Here's the drawing with two shaded views (mm, measured from the low corner). I have some questions. A direction names the side the tool comes from. Coordinates: 2 decimals unless noted, no trailing zeros. Write each loop counter-clockwise with the first axis right and the second up, starting at its lowest first coordinate (ties: lowest second). Pieces come first, ordered by that corner, then holes. Notation, with made-up numbers: (60, 40.5) -> (110, 40.5) arc R27 ccw to (110, 66.5) -> close; hole circle Ø3 at (30, 71). An arc over 180 degrees is marked (long way). Use one line per item in the form item = value.
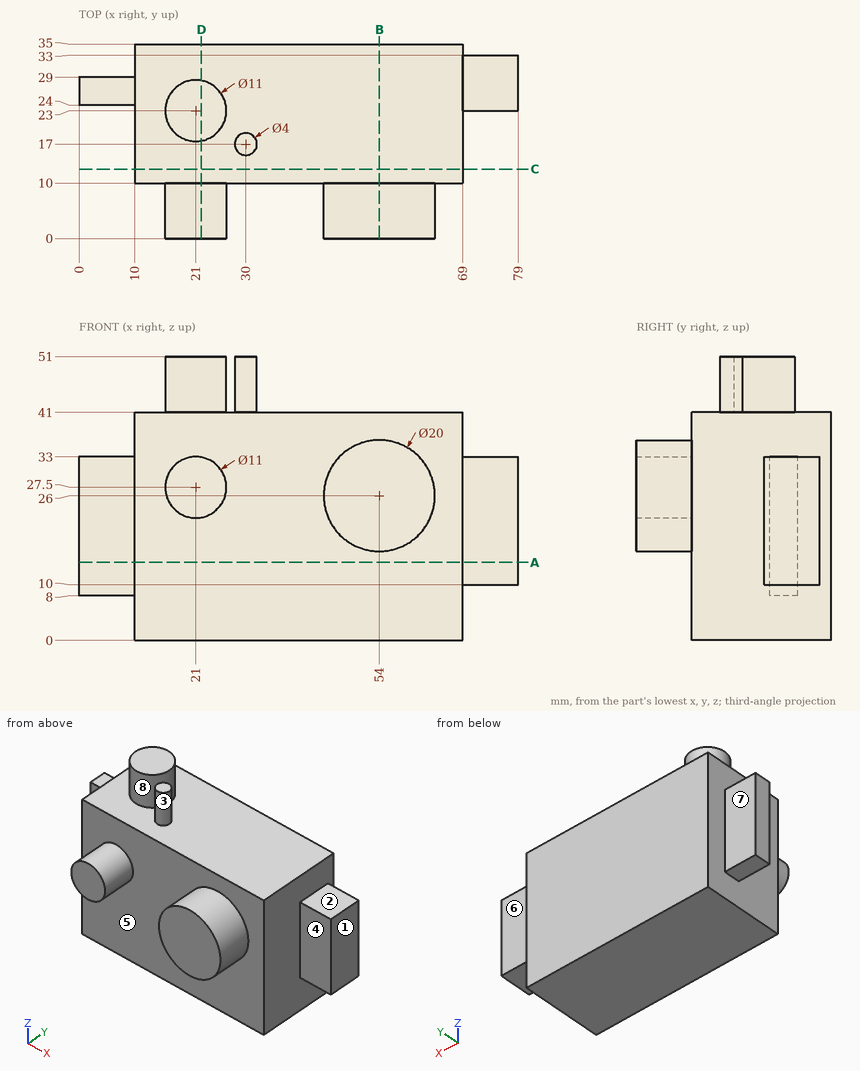
Q1. Suppose I cut it at B-B (x = 54). Write out the boundary of the cut face in (y, z), then the cut area to 4 significant figures.
Return value:
outline = (0, 16) -> (10, 16) -> (10, 0) -> (35, 0) -> (35, 41) -> (10, 41) -> (10, 36) -> (0, 36) -> close
area = 1,225 mm2
Q2. Suppose I cut it at A-A (z = 14). Write out the boundary of the cut face in (x, y).
Return value:
outline = (0, 24) -> (10, 24) -> (10, 10) -> (69, 10) -> (69, 23) -> (79, 23) -> (79, 33) -> (69, 33) -> (69, 35) -> (10, 35) -> (10, 29) -> (0, 29) -> close
Q3. Thinking about a two-plate mould opening in X: for the marked faces 1, 2 and 3, which applies, released by +X, released by -X, zero draft, split by the parting line, or undercut?
Return value:
face_1 = released by +X
face_2 = zero draft
face_3 = undercut
Q4. If I drill on line 1 (X direction, y = 19.5, z = 37.5); line 2 (Y direction, x = 28, z = 29.5); line 3 (Z direction, x = 11.5, y = 29), over which ranges is the centre line in solid material (lowest first)? Write a range as from..to.
Return value:
line_1 = 10..69
line_2 = 10..35
line_3 = 0..41
Q5. For the marked faces 4, 5, 6, 7 and 8, which set-ups out of +Z, -Z, +X, -X, +Y, -Y let a thin tool reach every point of the face, with its end or its side?
Return value:
face_4 = +Z, -Z, +X, -Y
face_5 = -Y
face_6 = +Z, -Z, +X, +Y
face_7 = +Z, -Z, -X, +Y
face_8 = +Z
Q6. Suppose I cut it at C-C (y = 12.5). Write out the boundary of the cut face in (x, z).
Return value:
outline = (10, 0) -> (69, 0) -> (69, 41) -> (10, 41) -> close
Q7. Suppose I cut it at D-D (x = 22). Write out the boundary of the cut face in (y, z).
Return value:
outline = (0, 22.09) -> (10, 22.09) -> (10, 0) -> (35, 0) -> (35, 41) -> (28.41, 41) -> (28.41, 51) -> (17.59, 51) -> (17.59, 41) -> (10, 41) -> (10, 32.91) -> (0, 32.91) -> close
Q8. Will these pins go through, and if not, where does the flat tip stop? pin 1 (2.5 mm diameter, centred on x = 6.5, y = 25.5, fed in from +Z); pin 2 (3 mm diameter, centred on y = 10.5, z = 10, fed in from -X); pin 3 (3 mm diameter, centred on x = 74, y = 29, fed in from -Z); pin 4 (12.5 mm diameter, centred on y = 20, z = 18.5, fed in from +X).
Return value:
pin_1 = 33
pin_2 = 10
pin_3 = 10
pin_4 = 79
